```python
from build123d import *

# Parameters (mm, degrees)
SKETCH_1_W                = 50
SKETCH_1_H                = 50
EXTRUDE_2_DEPTH           = 100
FILLET_4_R                = 3
SKETCH_3_W                = 44
SKETCH_3_H                = 44
CUT_EXTRUDE_4_DEPTH       = 80
SKETCH_3_4_W              = 44
SKETCH_3_4_H              = 44
EXTRUDE_4_DEPTH           = 20
SKETCH_7_W                = 44
SKETCH_7_H                = 20
CUT_EXTRUDE_5_DEPTH       = 20
SKETCH_7_2_W              = 44
SKETCH_7_2_H              = 20
EXTRUDE_5_DEPTH           = 5
SKETCH_9_W                = 44
SKETCH_9_H                = 20
CUT_EXTRUDE_6_DEPTH       = 20
SKETCH_9_2_W              = 44
SKETCH_9_2_H              = 20
EXTRUDE_6_DEPTH           = 3
CUT_EXTRUDE_7_DEPTH       = 5
CUT_EXTRUDE_7_DEPTH_BACK  = 5
SKETCH_15_W               = 44
SKETCH_15_H               = 20
CUT_EXTRUDE_9_DEPTH       = 41
SKETCH_15_2_W             = 44
SKETCH_15_2_H             = 20
EXTRUDE_7_DEPTH           = 15
SKETCH_15_3_W             = 44
SKETCH_15_3_H             = 20
CUT_EXTRUDE_10_DEPTH      = 10
SKETCH_16_W               = 44
SKETCH_16_H               = 20
CUT_EXTRUDE_11_DEPTH      = 30
SKETCH_16_2_W             = 44
SKETCH_16_2_H             = 20
EXTRUDE_8_DEPTH           = 13
SKETCH_16_3_W             = 44
SKETCH_16_3_H             = 20
CUT_EXTRUDE_12_DEPTH      = 10
CUT_EXTRUDE_17_DEPTH      = 40
CUT_EXTRUDE_18_DEPTH      = 5
CUT_EXTRUDE_18_DEPTH_BACK = 4
SKETCH_21_W               = 20
SKETCH_21_H               = 15
CUT_EXTRUDE_19_DEPTH      = 44
SKETCH_23_W               = 32
SKETCH_23_H               = 72
CUT_EXTRUDE_20_DEPTH      = 44
SKETCH_25_W               = 30
SKETCH_25_H               = 35
CUT_EXTRUDE_21_DEPTH      = 40
FILLET_5_R                = 3
FILLET_6_R                = 3


with BuildPart() as part:
    # 草图1 → 凸台-拉伸2 (new body)
    with BuildSketch(Plane(origin=(0, 0, 0), x_dir=(1, 0, 0), z_dir=(0, 1, 0))):
        Rectangle(SKETCH_1_W, SKETCH_1_H)
    extrude(amount=EXTRUDE_2_DEPTH)

    # 圆角4
    fillet_4_edges = [part.edges().sort_by_distance(p)[0] for p in [
        (-25, 50, 25),
        (-25, 50, -25),
        (25, 50, -25),
        (25, 50, 25),
    ]]
    fillet(fillet_4_edges, radius=FILLET_4_R)

    # 草图3 → 切除-拉伸4 (cut)
    with BuildSketch(Plane(origin=(0, 0, 0), x_dir=(1, 0, 0), z_dir=(0, 1, 0))):
        Rectangle(SKETCH_3_W, SKETCH_3_H)
    extrude(amount=CUT_EXTRUDE_4_DEPTH, mode=Mode.SUBTRACT)

    # 草图3<4> → 凸台-拉伸4 (add)
    with BuildSketch(Plane(origin=(0, 0, 0), x_dir=(1, 0, 0), z_dir=(0, 1, 0))):
        Rectangle(SKETCH_3_4_W, SKETCH_3_4_H)
    extrude(amount=EXTRUDE_4_DEPTH)

    # 草图7 → 切除-拉伸5 (cut)
    with BuildSketch(Plane(origin=(0, 0, 0), x_dir=(1, 0, 0), z_dir=(0, 1, 0))):
        with Locations((0, -12)):
            Rectangle(SKETCH_7_W, SKETCH_7_H)
    extrude(amount=CUT_EXTRUDE_5_DEPTH, mode=Mode.SUBTRACT)

    # 草图7<2> → 凸台-拉伸5 (add)
    with BuildSketch(Plane(origin=(0, 0, 0), x_dir=(1, 0, 0), z_dir=(0, 1, 0))):
        with Locations((0, -12)):
            Rectangle(SKETCH_7_2_W, SKETCH_7_2_H)
    extrude(amount=EXTRUDE_5_DEPTH)

    # 草图9 → 切除-拉伸6 (cut)
    with BuildSketch(Plane(origin=(0, 0, 0), x_dir=(1, 0, 0), z_dir=(0, 1, 0))):
        with Locations((0, 12)):
            Rectangle(SKETCH_9_W, SKETCH_9_H)
    extrude(amount=CUT_EXTRUDE_6_DEPTH, mode=Mode.SUBTRACT)

    # 草图9<2> → 凸台-拉伸6 (add)
    with BuildSketch(Plane(origin=(0, 0, 0), x_dir=(1, 0, 0), z_dir=(0, 1, 0))):
        with Locations((0, 12)):
            Rectangle(SKETCH_9_2_W, SKETCH_9_2_H)
    extrude(amount=EXTRUDE_6_DEPTH)

    # 草图10 → 切除-拉伸7 (cut, two sides: drawn at the far end of the back side and taken through both)
    with BuildSketch(Plane.XY.offset(-CUT_EXTRUDE_7_DEPTH_BACK)):
        with BuildLine():
            Line((-11.15, 18), (-11.15, 12))
            ThreePointArc((-11.15, 12), (-12, 11.15), (-12.85, 12))
            Line((-12.85, 12), (-12.85, 18))
            ThreePointArc((-12.85, 18), (-12, 18.85), (-11.15, 18))
        make_face()
        with BuildLine():
            Line((12.85, 18), (12.85, 12))
            ThreePointArc((12.85, 12), (12, 11.15), (11.15, 12))
            Line((11.15, 12), (11.15, 18))
            ThreePointArc((11.15, 18), (12, 18.85), (12.85, 18))
        make_face()
    extrude(amount=CUT_EXTRUDE_7_DEPTH + CUT_EXTRUDE_7_DEPTH_BACK, mode=Mode.SUBTRACT)

    # 草图15 → 切除-拉伸9 (cut)
    with BuildSketch(Plane(origin=(0, 110, 0), x_dir=(1, 0, 0), z_dir=(0, 1, 0))):
        with Locations((0, -12)):
            Rectangle(SKETCH_15_W, SKETCH_15_H)
    extrude(amount=-CUT_EXTRUDE_9_DEPTH, mode=Mode.SUBTRACT)

    # 草图15<2> → 凸台-拉伸7 (add)
    with BuildSketch(Plane(origin=(0, 110, 0), x_dir=(1, 0, 0), z_dir=(0, 1, 0))):
        with Locations((0, -12)):
            Rectangle(SKETCH_15_2_W, SKETCH_15_2_H)
    extrude(amount=-EXTRUDE_7_DEPTH)

    # 草图15<3> → 切除-拉伸10 (cut)
    with BuildSketch(Plane(origin=(0, 110, 0), x_dir=(1, 0, 0), z_dir=(0, 1, 0))):
        with Locations((0, -12)):
            Rectangle(SKETCH_15_3_W, SKETCH_15_3_H)
    extrude(amount=-CUT_EXTRUDE_10_DEPTH, mode=Mode.SUBTRACT)

    # 草图16 → 切除-拉伸11 (cut)
    with BuildSketch(Plane(origin=(0, 110, 0), x_dir=(1, 0, 0), z_dir=(0, 1, 0))):
        with Locations((-0.197660017, 12)):
            Rectangle(SKETCH_16_W, SKETCH_16_H)
    extrude(amount=-CUT_EXTRUDE_11_DEPTH, mode=Mode.SUBTRACT)

    # 草图16<2> → 凸台-拉伸8 (add)
    with BuildSketch(Plane(origin=(0, 110, 0), x_dir=(1, 0, 0), z_dir=(0, 1, 0))):
        with Locations((-0.197660017, 12)):
            Rectangle(SKETCH_16_2_W, SKETCH_16_2_H)
    extrude(amount=-EXTRUDE_8_DEPTH)

    # 草图16<3> → 切除-拉伸12 (cut)
    with BuildSketch(Plane(origin=(0, 110, 0), x_dir=(1, 0, 0), z_dir=(0, 1, 0))):
        with Locations((-0.197660017, 12)):
            Rectangle(SKETCH_16_3_W, SKETCH_16_3_H)
    extrude(amount=-CUT_EXTRUDE_12_DEPTH, mode=Mode.SUBTRACT)

    # 草图11 → 切除-拉伸17 (cut)
    with BuildSketch(Plane(origin=(0, 110, 0), x_dir=(1, 0, 0), z_dir=(0, 1, 0))):
        with BuildLine():
            Line((-16.15, 17), (-16.15, -13))
            ThreePointArc((-16.15, -13), (-17, -13.85), (-17.85, -13))
            Line((-17.85, -13), (-17.85, 17))
            ThreePointArc((-17.85, 17), (-17, 17.85), (-16.15, 17))
        make_face()
        with BuildLine():
            Line((17.85, 17), (17.85, -13))
            ThreePointArc((17.85, -13), (17, -13.85), (16.15, -13))
            Line((16.15, -13), (16.15, 17))
            ThreePointArc((16.15, 17), (17, 17.85), (17.85, 17))
        make_face()
    extrude(amount=-CUT_EXTRUDE_17_DEPTH, mode=Mode.SUBTRACT)

    # 草图20 → 切除-拉伸18 (cut, two sides: drawn at the far end of the back side and taken through both)
    with BuildSketch(Plane.XY.offset(-CUT_EXTRUDE_18_DEPTH_BACK)):
        with BuildLine():
            Line((-11.15, 90), (-11.15, 82))
            ThreePointArc((-11.15, 82), (-12, 81.15), (-12.85, 82))
            Line((-12.85, 82), (-12.85, 90))
            ThreePointArc((-12.85, 90), (-12, 90.85), (-11.15, 90))
        make_face()
        with BuildLine():
            Line((12.85, 90), (12.85, 82))
            ThreePointArc((12.85, 82), (12, 81.15), (11.15, 82))
            Line((11.15, 82), (11.15, 90))
            ThreePointArc((11.15, 90), (12, 90.85), (12.85, 90))
        make_face()
    extrude(amount=CUT_EXTRUDE_18_DEPTH + CUT_EXTRUDE_18_DEPTH_BACK, mode=Mode.SUBTRACT)

    # 草图21 → 切除-拉伸19 (cut)
    with BuildSketch(Plane(origin=(0, 110, 0), x_dir=(1, 0, 0), z_dir=(0, 1, 0))):
        with Locations((-0.808809207, 12.5)):
            Rectangle(SKETCH_21_W, SKETCH_21_H)
    extrude(amount=-CUT_EXTRUDE_19_DEPTH, mode=Mode.SUBTRACT)

    # 草图23 → 切除-拉伸20 (cut)
    with BuildSketch(Plane.XY):
        with Locations((0, 56)):
            Rectangle(SKETCH_23_W, SKETCH_23_H)
    extrude(amount=-CUT_EXTRUDE_20_DEPTH, mode=Mode.SUBTRACT)

    # 草图25 → 切除-拉伸21 (cut)
    with BuildSketch(Plane.XY):
        with Locations((0, 60.5)):
            Rectangle(SKETCH_25_W, SKETCH_25_H)
    extrude(amount=CUT_EXTRUDE_21_DEPTH, mode=Mode.SUBTRACT)

    # 圆角5
    fillet_5_edges = [part.edges().sort_by_distance(p)[0] for p in [
        (-15, 78, 23.5),
        (-15, 43, 23.5),
        (15, 43, 23.5),
        (15, 78, 23.5),
    ]]
    fillet(fillet_5_edges, radius=FILLET_5_R)

    # 圆角6
    fillet_6_edges = [part.edges().sort_by_distance(p)[0] for p in [
        (-10.808809207, 98.5, -5),
        (-10.808809207, 98.5, -20),
        (9.191190793, 98.5, -20),
        (9.191190793, 98.5, -5),
    ]]
    fillet(fillet_6_edges, radius=FILLET_6_R)


solid = part.part
```
Here's how the part is built. I have some questions about the finished solid (model axes, mm). A direction names the side the tool comes from. Give positions to 0.01 mm unless a question says otherwise; leave off trailing zeros. Write each loop counter-clockwise with the first axis right and the second up, starting at its lowest first coordinate (ties: lowest second). Pieces come first, ordered by that corner, then holes. Notation, with made-up numbers: M 25,-20 L 32,-20 A28 ccw 32,10 Z; hole C -28,-8 d7. An arc over 180 degrees is marked long. Put each result on its own line as item: value. Start each with the question number.
Item 1: On a 3-axis mill with a long thin cutter (end or side, diameter ignored), from which of +Z, -Z, +X, -X, +Y, -Y can I reach the whole of each face in a straight line? I mean faces 1 (the flat face through (-16, 55, -23)), 2 (the cylindrical face through (14.1, 77.14, 23.52)), 3 (the flat face through (-11.15, 15, 0)), 4 (the cylindrical face through (8.336, 98.479, -19.098)). Say none if no direction works.
Item 2: Thinking about a two-plate mould opening in Y: for faces 5 (the flat face through (0, 80, 1)), 6 (the cylindrical face through (24.1, 50.7, 24.14)), which applies, +Y half, -Y half, draft (parallel to the pull), parting line (faces both ways), or undercut?
Item 3: If we section it at B-B, the plane x = -2: Count the separate pieces of the cut face and the enclosed holes in it, then the cut area to 3 significant figures.
Item 4: If we section it at C-C, the plane z = 7.5: Write out the boundary of the cut face in (x, y), then the cut area to 3 significant figures.
Item 5: If we section it at D-D, the plane x = -19: Write out the boundary of the cut face in (y, z).
Item 6: If we section it at A-A, the plane y = 16.5: Write out the boundary of the cut face in (x, z).
Item 7: I need wall thicknesses on L1, parallel to Z at x = 11, y = 11; L2, parallel to Z at x = 16.5, y = 56.5. Which ranges of each line are inside material? Lowest first, please. Write a range as from..to.
Values:
1. face 1: -Z
1. face 2: +Z, -Z
1. face 3: none
1. face 4: +Y
2. face 5: undercut
2. face 6: draft
3. separate pieces: 3
3. enclosed holes: 0
3. area: 690 mm²
4. outline: M -25,0 L 25,0 L 25,100 L 17.85,100 L 17.85,95 L 22,95 L 22,5 L -22,5 L -22,95 L -17.85,95 L -17.85,100 L -25,100 Z; M -16.15,95 L 16.15,95 L 16.15,100 L -16.15,100 Z
4. area: 1,020 mm²
5. outline: M 0,-25 L 100,-25 L 100,25 L 0,25 Z; hole M 3,-22 L 97,-22 L 97,-2 L 80,-2 L 80,2 L 95,2 L 95,22 L 5,22 L 5,2 L 20,2 L 20,-2 L 3,-2 Z
6. outline: M -25,-22 A3 ccw -22,-25 L 22,-25 A3 ccw 25,-22 L 25,22 A3 ccw 22,25 L -22,25 A3 ccw -25,22 Z; M -11.15,-2 L 11.15,-2 L 11.15,2 L -11.15,2 Z; hole M -22,-22 L 22,-22 L 22,-2 L 12.85,-2 L 12.85,2 L 22,2 L 22,22 L -22,22 L -22,2 L -12.85,2 L -12.85,-2 L -22,-2 Z
7. L1: -25..-22, -2..2, 22..25
7. L2: -25..-22, 22..25
